from build123d import *

# Parameters (mm, degrees)
F1_DEPTH = 6.35
F2_DEPTH = 7.9375
F3_DEPTH = 1.5875


# Not quite as in the source:
# - a length typed as a fraction of an inch, garbled in the dataset ("3 / 203.2 mm" for 3/8 in), is restored


with BuildPart() as f1:
    # F0 (on Top) → F1 (new body)
    with BuildSketch(Plane.XY):
        with BuildLine():
            ThreePointArc((-24.0030003875, -9.8155226706), (-14.8352444226, -3.5452855547), (-11.3030003875, 6.9849981546))
            ThreePointArc((-11.3030003875, 6.9849981546), (-39.2957840969, 20.9152541196), (-33.5280003875, -9.8155226706))
            Line((-33.5280003875, -9.8155226706), (-33.5280003875, 6.9849981546))
            Line((-33.5280003875, 6.9849981546), (-24.0030003875, 6.9849981546))
            Line((-24.0030003875, 6.9849981546), (-24.0030003875, -9.8155226706))
        make_face()
    extrude(amount=F1_DEPTH)

    # F0 (on Top) → F2 (join)
    with BuildSketch(Plane.XY):
        with BuildLine():
            Line((-33.5280003875, 6.9849981546), (-33.5280003875, -9.8155226706))
            ThreePointArc((-33.5280003875, -9.8155226706), (-28.7655003875, -10.4775018454), (-24.0030003875, -9.8155226706))
            Line((-24.0030003875, -9.8155226706), (-24.0030003875, 6.9849981546))
            Line((-24.0030003875, 6.9849981546), (-33.5280003875, 6.9849981546))
        make_face()
        with BuildLine():
            ThreePointArc((-24.0030003875, -9.8155226706), (-28.7655003875, -10.4775018454), (-33.5280003875, -9.8155226706))
            Line((-33.5280003875, -9.8155226706), (-33.5280003875, -43.8150018454))
            ThreePointArc((-33.5280003875, -43.8150018454), (-28.7655003875, -48.5775018454), (-24.0030003875, -43.8150018454))
            Line((-24.0030003875, -43.8150018454), (-24.0030003875, -9.8155226706))
        make_face()
    extrude(amount=F2_DEPTH)

    # F0 (on Top) → F3 (join)
    with BuildSketch(Plane.XY):
        with BuildLine():
            ThreePointArc((-24.0030003875, -9.8155226706), (-28.7655003875, -10.4775018454), (-33.5280003875, -9.8155226706))
            Line((-33.5280003875, -9.8155226706), (-33.5280003875, -43.8150018454))
            ThreePointArc((-33.5280003875, -43.8150018454), (-28.7655003875, -48.5775018454), (-24.0030003875, -43.8150018454))
            Line((-24.0030003875, -43.8150018454), (-24.0030003875, -9.8155226706))
        make_face()
        with BuildLine():
            Line((-33.5280003875, 6.9849981546), (-33.5280003875, -9.8155226706))
            ThreePointArc((-33.5280003875, -9.8155226706), (-28.7655003875, -10.4775018454), (-24.0030003875, -9.8155226706))
            Line((-24.0030003875, -9.8155226706), (-24.0030003875, 6.9849981546))
            Line((-24.0030003875, 6.9849981546), (-33.5280003875, 6.9849981546))
        make_face()
    extrude(amount=-F3_DEPTH)


solid = f1.part
Design review of the part built by this model. Coordinates are the model's own, in mm. A direction names the side the tool comes from. Round coordinates to 2 decimals unless told otherwise and drop trailing zeros. Write each loop counter-clockwise with the first axis right and the second up, starting at its lowest first coordinate (ties: lowest second). Pieces come first, ordered by that corner, then holes.
Item 1: Consider section C-C on y = -28. Give the boundary of the cut face in (x, z), and give its area (3 significant figures).
Item 2: For pin 1 Ø5 at (x, z) = (-16.5, 2.5) entering from -Y; pin 2 Ø1 at (y, z) = (-26.5, 3.5) entering from +X; pin 3 Ø0.8 at (x, z) = (-27.5, -1) entering from +Y (3 decimals), all flat-tipped, find the tip position at first contact; note any pin that passes through.
Item 3: For faces 1 (the flat face through (-29, 6.985, 7)), 2 (the cylindrical face through (-28.87, -48.576, 3.242)), 3 (the flat face through (-29, 6.985, -1)), list the 3-axis set-ups (+Z, -Z, +X, -X, +Y, -Y) from which the entire face can be reached by the end or side of a thin tool; tool diameter is ignored.
Item 4: Consider section A-A on z = 3.5. Give the boundary of the cut face in (x, y) (1 decimal).
Item 5: Wall thickness on L1, parallel to Z at x = -19, y = 10.5; L2, parallel to X at y = -20, z = -0.25; L3, parallel to X at y = 11.5, z = 2.5: over which ranges is each line inside the solid? List them lowest first.
Check values:
1. outline: (-33.53, -1.59) - (-24, -1.59) - (-24, 7.94) - (-33.53, 7.94) - close
1. area: 90.7 mm2
2. pin 1: stops at y = -7.49
2. pin 2: stops at x = -24
2. pin 3: stops at y = 6.985
3. face 1: +Z, +X, -X, +Y
3. face 2: +Z, -Z, -Y
3. face 3: -Z, +X, -X, +Y
4. outline: (-33.5, -43.8) arc R4.8 ccw to (-24, -43.8) - (-24, -9.8) arc R17.5 ccw (long way) to (-33.5, -9.8) - close
5. L1: z = 0 to 6.35
5. L2: x = -33.53 to -24
5. L3: x = -45.63 to -11.9
